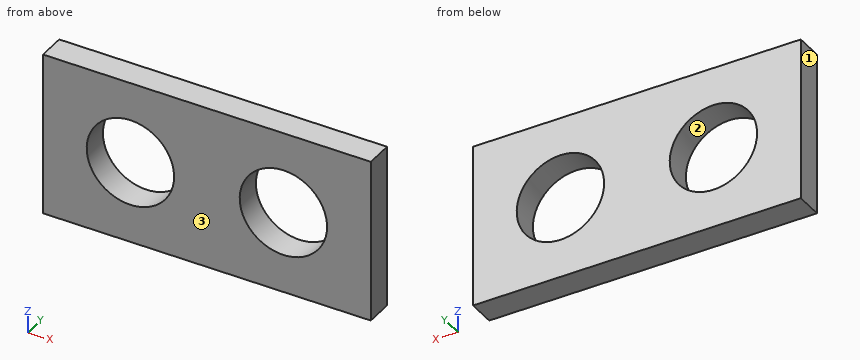
from build123d import *

# Parameters (mm, degrees)
SKETCH2_W               = 30
SKETCH2_H               = 15
BOSS_EXTRUDE1_DEPTH     = 2.5
CUT_EXTRUDE1_DEPTH      = 34.634060118
CUT_EXTRUDE1_DEPTH_BACK = 34.634060118
SKETCH4_R               = 4


with BuildPart() as part:
    # Sketch2 → Boss-Extrude1 (new body)
    with BuildSketch(Plane(origin=(0, 0, 0), x_dir=(1, 0, 0), z_dir=(0, 1, 0))):
        with Locations((15, 7.5)):
            Rectangle(SKETCH2_W, SKETCH2_H)
    extrude(amount=BOSS_EXTRUDE1_DEPTH)

    # Sketch4 → Cut-Extrude1 (cut, two sides: drawn at the far end of the back side and taken through both)
    with BuildSketch(Plane(origin=(0, 2.5, 0), x_dir=(1, 0, 0), z_dir=(0, 1, 0)).offset(-CUT_EXTRUDE1_DEPTH_BACK)):
        with Locations(Location((22, 7.5, 0), (0, 0, 270))):
            Circle(SKETCH4_R)
        with Locations(Location((8, 7.5, 0), (0, 0, 270))):
            Circle(SKETCH4_R)
    extrude(amount=CUT_EXTRUDE1_DEPTH + CUT_EXTRUDE1_DEPTH_BACK, mode=Mode.SUBTRACT)


solid = part.part
Design review of the part built by this model. Coordinates are the model's own, in mm. Face numbers are marked on the shaded views. Give positions to 0.01 mm unless a question says otherwise; leave off trailing zeros. Write each loop counter-clockwise with the first axis right and the second up, starting at its lowest first coordinate (ties: lowest second). Pieces come first, ordered by that corner, then holes. Notation, with made-up numbers: M -6.75,19.25 L 39.25,19.25 A13 ccw 39.25,43.25 Z; hole C 55,40.5 d2. An arc over 180 degrees is marked long. Answer as a JSON object with one key per item and string values. Group by question number.
1) For line 1 along X through (y, z) = (1.75, -7.5); line 2 along Z through (x, y) = (8, 1.3); line 3 along X through (y, z) = (1.6, -10.25), list the stretches that pass through material, from the lowest coordinate up.
2) We need section B-B (x = 8). Give the boundary of the cut face in (y, z).
3) We need section A-A (z = -7.5). Give the boundary of the cut face in (x, y).
4) We need section C-C (y = 0.5). Give the boundary of the cut face in (x, z), and give its area (3 significant figures).
5) Clearance check with flat-ended pins moving along their axes: pin 1 Ø9 at (x, z) = (22, -7.5) entering from -Y; pin 2 Ø6.5 at (x, z) = (8, -7.5) entering from -Y. State where each tip first meets the part, or that it passes through.
6) We need section D-D (z = -10.5). Give the boundary of the cut face in (x, y), and give its area (3 significant figures).
7) Mouldability with a two-part tool opening along X and no side actions: class the marked faces 1, 2 and 3 as released by +X, released by -X, zero draft, split by the parting line, or undercut.
Answer key:
{
 "1": {"line 1": "x = 0 to 4, 12 to 18, 26 to 30", "line 2": "z = -15 to -11.5, -3.5 to 0", "line 3": "x = 0 to 5.1, 10.9 to 19.1, 24.9 to 30"},
 "2": {"outline": "M 0,-15 L 2.5,-15 L 2.5,-11.5 L 0,-11.5 Z; M 0,-3.5 L 2.5,-3.5 L 2.5,0 L 0,0 Z"},
 "3": {"outline": "M 0,0 L 4,0 L 4,2.5 L 0,2.5 Z; M 12,0 L 18,0 L 18,2.5 L 12,2.5 Z; M 26,0 L 30,0 L 30,2.5 L 26,2.5 Z"},
 "4": {"outline": "M 0,-15 L 30,-15 L 30,0 L 0,0 Z; hole C 8,-7.5 d8; hole C 22,-7.5 d8", "area": "349 mm²"},
 "5": {"pin 1": "stops at y = 0", "pin 2": "passes through"},
 "6": {"outline": "M 0,0 L 5.35,0 L 5.35,2.5 L 0,2.5 Z; M 10.65,0 L 19.35,0 L 19.35,2.5 L 10.65,2.5 Z; M 24.65,0 L 30,0 L 30,2.5 L 24.65,2.5 Z", "area": "48.5 mm²"},
 "7": {"face 1": "released by -X", "face 2": "undercut", "face 3": "zero draft"}
}
